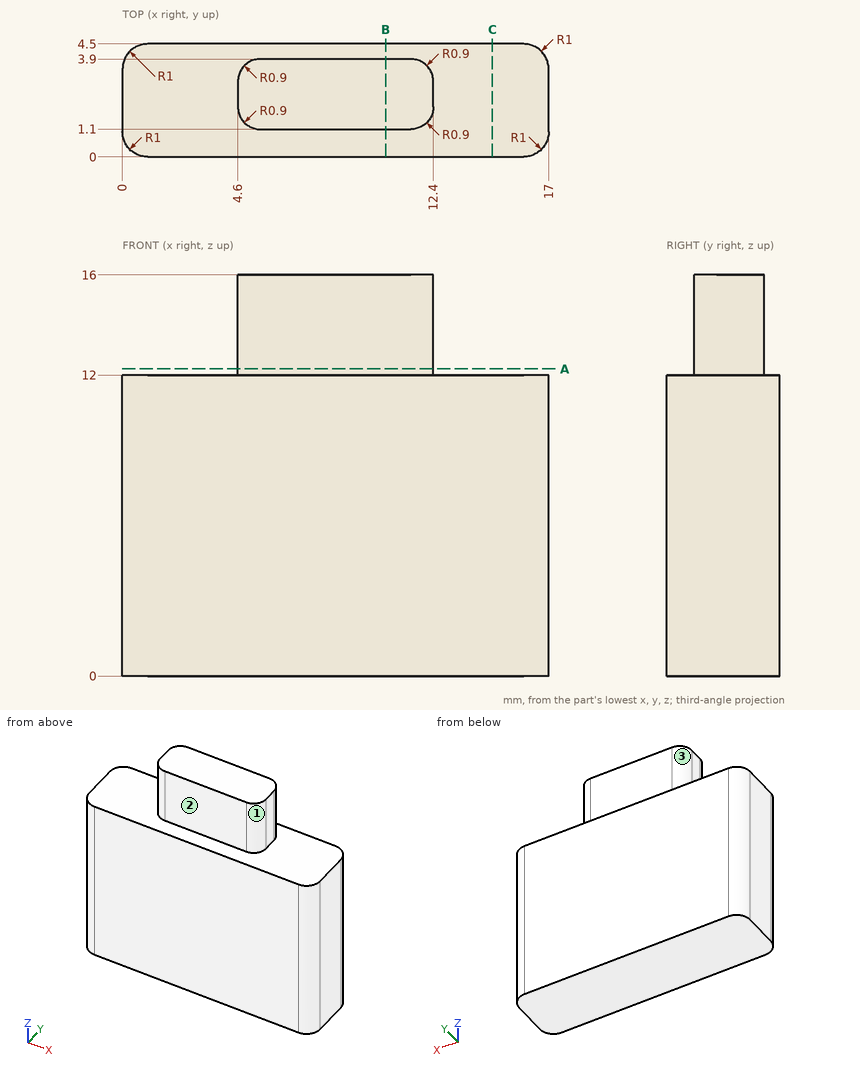
Study the drawing (mm; zero at the part's minimum x, y, z) and answer. A direction names the side the tool comes from. Coordinates: 2 decimals unless noted, no trailing zeros. Order: outer loops, then holes, each group sorted by start corner. A loop starts at its lowest first (then second) coordinate and runs counter-clockwise, first axis right, second up. Notation, with made-up numbers: M 25,53 L 40,53 A25 cw 40,77 Z; hole C 36,78 d11. An arc over 180 degrees is marked long. Answer as a JSON object with one key per item and string values. Group by question number.
1. Section B-B on x = 10.5 is taken. Write down the section's boundary in (y, z), then the cut area to 3 significant figures.
2. Flat-ended cylindrical pins translate along their axes: P1, Ø0.5, axis at y = 2.5, z = 13, coming from the -X side; P2, Ø0.8, axis at y = 2.5, z = 13.5, coming from the +X side; P3, Ø1.2, axis at x = 7, z = 13.5, coming from the +Y side. Find the tip coordinate at first contact, or state that the pin passes through.
3. Section A-A on z = 12.25 is taken. Write down the section's boundary in (x, y), then the cut area to 3 significant figures.
4. Straight lines are drawn through the part: line 1 (Z direction, x = 12.5, y = 0.75); line 2 (X direction, y = 2.75, z = 15.5); line 3 (Y direction, x = 8.75, z = 15.25). For each, find the intervals that lie inside material, in ascending order.
5. Section C-C on x = 14.75 is taken. Write down the section's boundary in (y, z).
6. A tool of negligible diameter and unlimited length cuts with its end or side. For the marked faces 1, 2 and 3, from which of +Z, -Z, +X, -X, +Y, -Y can it reach the whole face along a straight path? Write none if from no direction.
Values follow:
{
 "1": {"outline": "M 0,0 L 4.5,0 L 4.5,12 L 3.9,12 L 3.9,16 L 1.1,16 L 1.1,12 L 0,12 Z", "area": "65.2 mm2"},
 "2": {"P1": "x = 4.6", "P2": "x = 12.4", "P3": "y = 3.9"},
 "3": {"outline": "M 4.6,2 A0.9 ccw 5.5,1.1 L 11.5,1.1 A0.9 ccw 12.4,2 L 12.4,3 A0.9 ccw 11.5,3.9 L 5.5,3.9 A0.9 ccw 4.6,3 Z", "area": "21.1 mm2"},
 "4": {"line 1": "0 to 12", "line 2": "4.6 to 12.4", "line 3": "1.1 to 3.9"},
 "5": {"outline": "M 0,0 L 4.5,0 L 4.5,12 L 0,12 Z"},
 "6": {"face 1": "+Z, +X, -Y", "face 2": "+Z, +X, -X, -Y", "face 3": "+Z, -X, +Y"}
}
